Verification items for the finished model (mm, model axes). Face numbers are marked on the shaded views. A direction names the side the tool comes from. Coordinates: 2 decimals unless noted, no trailing zeros. Write each loop counter-clockwise with the first axis right and the second up, starting at its lowest first coordinate (ties: lowest second). Pieces come first, ordered by that corner, then holes. Notation, with made-up numbers: (38, -14) - (53, -14) arc R24 cw to (53, 23) - close; hole circle Ø9 at (44, 42). An arc over 180 degrees is marked (long way). Use one line per item in the form item = value. Start each with the question number.
(1) Gauge pin test, flat ends, axial feed: pin 1 Ø8 at (x, y) = (49, 57) entering from -Z; pin 2 Ø4.5 at (x, z) = (3, 1.5) entering from +Y; pin 3 Ø1 at (x, z) = (56, 5) entering from +Y; pin 4 Ø2 at (y, z) = (26, 2.5) entering from +X. Record the tip position at first contact, or that the pin passes through.
(2) Material ranges on line 1 (Y direction, x = 21, z = 0.85); line 2 (X direction, y = 1, z = 8); line 3 (Y direction, x = 41.5, z = 1.5), recorded low to high. Write a range as [from, to].
(3) Sectioned sample at A-A (y = 11). Record the cut outline in (x, z), and give its area (3 significant figures).
(4) Tool access check on the marked faces 1 and 2. Record the directions out of +Z, -Z, +X, -X, +Y, -Y that give a thin tool (end or side, any length) a straight path to the whole face; none if there is none.
(5) Sectioned sample at B-B (x = 21). Record the cut outline in (y, z).
(6) Sectioned sample at D-D (y = 37.5). Record the cut outline in (x, z), and give its area (3 significant figures).
(7) Sectioned sample at C-C (x = 93). Record the cut outline in (y, z).
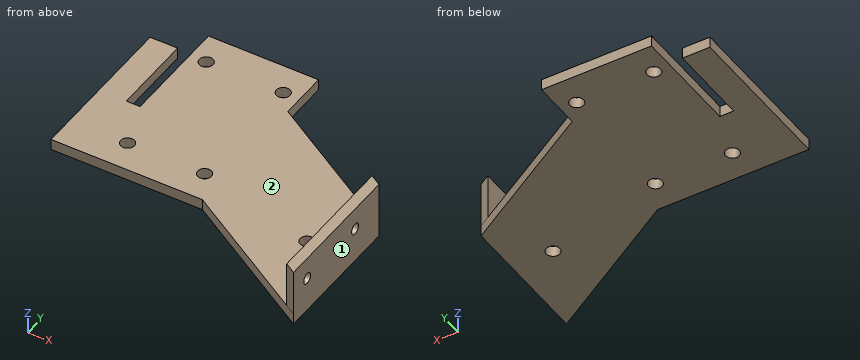
from build123d import *

# Parameters (mm, degrees)
SKETCH_1_R          = 2.5
EXTRUDE_1_DEPTH     = 4
EXTRUDE_2_DEPTH     = 16.7
SKETCH_3_R          = 2
CUT_EXTRUDE_1_DEPTH = 10
CUT_EXTRUDE_2_DEPTH = 10


with BuildPart() as part:
    # Эскиз1 → Бобышка-Вытянуть1 (new body)
    with BuildSketch(Plane.XY):
        Polygon((0, 0), (55, 0), (108, -32), (108, 0), (108, 18), (55, 50), (55, 68), (0, 68), align=None)
        with Locations((21, 57)):
            Circle(SKETCH_1_R, mode=Mode.SUBTRACT)
        with Locations((49, 57)):
            Circle(SKETCH_1_R, mode=Mode.SUBTRACT)
        with Locations((21, 11)):
            Circle(SKETCH_1_R, mode=Mode.SUBTRACT)
        with Locations((49, 11)):
            Circle(SKETCH_1_R, mode=Mode.SUBTRACT)
        with Locations((93, 0)):
            Circle(SKETCH_1_R, mode=Mode.SUBTRACT)
    extrude(amount=EXTRUDE_1_DEPTH)

    # Эскиз2 → Бобышка-Вытянуть2 (add)
    with BuildSketch(Plane.XY.offset(4)):
        Polygon((108, 18), (108, -32), (104, -29.58490566), (104, 20.41509434), align=None)
    extrude(amount=EXTRUDE_2_DEPTH)

    # Эскиз3 → Вырез-Вытянуть1 (cut)
    with BuildSketch(Plane(origin=(108, 0, 0), x_dir=(0, 0, -1), z_dir=(1, 0, 0))):
        with Locations((-12.7, 4)):
            Circle(SKETCH_3_R)
        with Locations((-12.7, -24)):
            Circle(SKETCH_3_R)
    extrude(amount=-CUT_EXTRUDE_1_DEPTH, mode=Mode.SUBTRACT)

    # Эскиз4 → Вырез-Вытянуть2 (cut)
    with BuildSketch(Plane.XY.offset(4)):
        Polygon((0, 68), (15, 68), (15, 58), (15, 28), (10, 28), (10, 58), (0, 58), align=None)
    extrude(amount=-CUT_EXTRUDE_2_DEPTH, mode=Mode.SUBTRACT)


solid = part.part
Answers below:
q1.pin_1 = 0
q1.pin_2 = 58
q1.pin_3 = through
q1.pin_4 = 96.41
q2.line_1 = [0, 8.5], [13.5, 54.5], [59.5, 68]
q2.line_2 = [104, 108]
q2.line_3 = [0, 68]
q3.outline = (0, 0) - (18.5, 0) - (18.5, 4) - (0, 4) - close; (23.5, 0) - (46.5, 0) - (46.5, 4) - (23.5, 4) - close; (51.5, 0) - (108, 0) - (108, 20.7) - (104, 20.7) - (104, 4) - (51.5, 4) - close
q3.area = 459 mm2
q4.face_1 = +Z, -Z, +X, +Y, -Y
q4.face_2 = +Z, -X, +Y, -Y
q5.outline = (0, 0) - (8.5, 0) - (8.5, 4) - (0, 4) - close; (13.5, 0) - (54.5, 0) - (54.5, 4) - (13.5, 4) - close; (59.5, 0) - (68, 0) - (68, 4) - (59.5, 4) - close
q6.outline = (0, 0) - (10, 0) - (10, 4) - (0, 4) - close; (15, 0) - (75.7, 0) - (75.7, 4) - (15, 4) - close
q6.area = 283 mm2
q7.outline = (-22.94, 0) - (-2.5, 0) - (-2.5, 4) - (-22.94, 4) - close; (2.5, 0) - (27.06, 0) - (27.06, 4) - (2.5, 4) - close
